from build123d import *

# Parameters (mm, degrees)
SKETCH1_R          = 16.5354
EXTRUDE1_DEPTH     = 53.848
CHAMFER1_SIZE      = 0.762
SKETCH6_R          = 15.6845
EXTRUDE2_DEPTH     = 5.969
SKETCH7_W          = 14.478
SKETCH7_H          = 10.31875
CUT_EXTRUDE4_DEPTH = 19.84248
HOLE1_D            = 5.0038
HOLE1_DEPTH        = 4.7498
CIRPATTERN1_COUNT  = 4


with BuildPart() as part:
    # Sketch1 → Extrude1 (new body)
    with BuildSketch(Plane.XY):
        Circle(SKETCH1_R)
    extrude(amount=EXTRUDE1_DEPTH)

    # Sketch2 → Cut-Revolve1 (revolve, cut)
    with BuildSketch(Plane(origin=(0, 0, 0), x_dir=(1, 0, 0), z_dir=(0, 1, 0)), mode=Mode.PRIVATE) as cut_revolve1_sk:
        Polygon((16.5354, -53.848), (16.5354, -39.9034), (15.2908, -41.148), (15.2908, -53.848), align=None)
    revolve(cut_revolve1_sk.sketch.rotate(Axis((0, 0, 0), (0, 0, 1)), 180), axis=Axis((0, 0, 0), (0, 0, 1)), mode=Mode.SUBTRACT)  # turned: the seam where the file's is

    # Sketch3 → Cut-Revolve2 (revolve, cut)
    with BuildSketch(Plane(origin=(0, 0, 0), x_dir=(1, 0, 0), z_dir=(0, 1, 0)), mode=Mode.PRIVATE) as cut_revolve2_sk:
        Polygon((15.2908, 0), (15.2908, -1.524), (16.5354, -2.7686), (16.5354, 0), align=None)
    revolve(cut_revolve2_sk.sketch.rotate(Axis((0, 0, 0), (0, 0, -1)), 180), axis=Axis((0, 0, 0), (0, 0, -1)), mode=Mode.SUBTRACT)  # turned: the seam where the file's is

    # S2D0002 → Cut-Revolve3 (revolve, cut)
    with BuildSketch(Plane(origin=(0, 0, 0), x_dir=(1, 0, 0), z_dir=(0, 1, 0))):
        Polygon((6.1849, -53.594), (9.525, -53.594), (9.525, -53.848), (0, -53.848), (0, -39.624), (4.9784, -39.624), (4.9784, -50.377393135), (5.642306865, -51.0413), align=None)
    revolve(axis=Axis((0, 0, 14.6685), (0, 0, -1)), mode=Mode.SUBTRACT)

    # Chamfer1
    chamfer1_edges = [part.edges().sort_by_distance(p)[0] for p in [
        (15.2908, 0, 53.848),
    ]]
    chamfer(chamfer1_edges, length=CHAMFER1_SIZE)

    # Sketch6 → Extrude2 (add)
    with BuildSketch(Plane(origin=(0, 0, 0), x_dir=(-1, 0, 0), z_dir=(0, 0, -1))):
        Circle(SKETCH6_R)
    extrude(amount=EXTRUDE2_DEPTH)

    # Sketch7 → Revolve1 (revolve)
    with BuildSketch(Plane(origin=(0, 0, 0), x_dir=(0, 0, -1), z_dir=(1, 0, 0)), mode=Mode.PRIVATE) as revolve1_sk:
        with Locations((13.208, -5.159375)):
            Rectangle(SKETCH7_W, SKETCH7_H)
    revolve(revolve1_sk.sketch.rotate(Axis((0, 0, 0), (0, 0, -1)), 270), axis=Axis((0, 0, 0), (0, 0, -1)))  # turned: the seam where the file's is

    # S2D0001 → Cut-Revolve5 (revolve, cut)
    with BuildSketch(Plane(origin=(0, 0, 0), x_dir=(1, 0, 0), z_dir=(0, 1, 0))):
        Polygon((3.2639, 18.511260017), (3.2639, 3.8608), (0, 3.8608), (0, 20.447), (4.3815, 20.447), align=None)
    revolve(axis=Axis((0, 0, 31.308359971), (0, 0, -1)), mode=Mode.SUBTRACT)

    # Sketch9 → Cut-Revolve6 (revolve, cut)
    with BuildSketch(Plane(origin=(0, 0, 0), x_dir=(0, -1, 0), z_dir=(1, 0, 0)), mode=Mode.PRIVATE) as cut_revolve6_sk:
        with BuildLine():
            Line((-10.31875, 13.0302), (-10.033, 13.7922))
            Line((-10.033, 13.7922), (-10.033, 19.431))
            ThreePointArc((-10.033, 19.431), (-9.932678675, 19.974796865), (-9.644922533, 20.447))
            Line((-9.644922533, 20.447), (-10.31875, 20.447))
            Line((-10.31875, 20.447), (-10.31875, 13.0302))
        make_face()
    revolve(cut_revolve6_sk.sketch.rotate(Axis((0, 0, -12.65936), (0, 0, -1)), 90), axis=Axis((0, 0, -12.65936), (0, 0, -1)), mode=Mode.SUBTRACT)  # turned: the seam where the file's is

    # Sketch13 → Cut-Extrude4 (cut, symmetric)
    with BuildSketch(Plane(origin=(0, 0, 0), x_dir=(1, 0, 0), z_dir=(0, 1, 0))):
        Polygon((8.5852, 20.447), (8.5852, 15.494), (10.033, 14.0462), (10.033, 20.447), align=None)
        Polygon((-8.5852, 20.447), (-8.5852, 15.494), (-10.033, 14.0462), (-10.033, 20.447), align=None)
    extrude(amount=CUT_EXTRUDE4_DEPTH, both=True, mode=Mode.SUBTRACT)

    # Hole1
    with Locations(Plane(origin=(-10.81222837, 10.81222837, 47.498), x_dir=(0.707106781, 0.707106781, 0), z_dir=(-0.707106781, 0.707106781, 0))):
        with Locations((0, 0)):
            hole1 = Hole(HOLE1_D / 2, depth=HOLE1_DEPTH)

    # CirPattern1: Hole1 ×4 about axis
    cirpattern1_axis = Axis((0, 0, 0), (0, 0, 1))
    for i in range(1, CIRPATTERN1_COUNT):
        add(hole1.rotate(cirpattern1_axis, i * 360 / CIRPATTERN1_COUNT), mode=Mode.SUBTRACT)


solid = part.part
Here's how the part is built. I have some questions about the finished solid (model axes, mm). A direction names the side the tool comes from. Round coordinates to 2 decimals unless told otherwise and drop trailing zeros. Write each loop counter-clockwise with the first axis right and the second up, starting at its lowest first coordinate (ties: lowest second). Pieces come first, ordered by that corner, then holes.
1. Suppose I cut it at B-B (z = 38). List the corners of the cut face in (x, y) for me.
2. For faces 4 (the cylindrical face through (-7.056, -13.566, 0.773)), 5 (the cylindrical face through (-14.125, 5.856, 47.201)), 6 (the flat face through (-10.2, -3.3, -5.969)), which set-ups out of +Z, -Z, +X, -X, +Y, -Y let a thin tool reach every point of the face, with its end or its side?
3. Suppose I cut it at D-D (z = -10). List the corners of the cut face in (x, y) for me.
4. Will these pins go through, and if not, where does the flat tip stop? pin 1 Ø12 at (x, z) = (9, -11.5) entering from -Y; pin 2 Ø6 at (x, y) = (9.5, -13) entering from -Z; pin 3 Ø3 at (x, y) = (2, 1) entering from +Z.
5. Suppose I cut it at C-C (x = 7). State how many separate pieces and enclosed holes the cut face has, and give its area (3 significant figures).
6. Suppose I cut it at A-A (z = 48.5). List the corners of the cut face in (x, y) for me, and give its area (3 significant figures).
7. If we mould it in two halves opening along X, with no side actions, what happens to faces 1 (the cylindrical face through (15.77, 4.97, 21.08)), 2 (the flat face through (9.14, -0.07, -14.94)), 3 (the cylindrical face through (4.749, -1.495, 45.076))? For each: released by +X, released by -X, zero draft, split by the parting line, or undercut.
8. I need wall thicknesses on L1, parallel to X at y = 9, z = 46; L2, parallel to X at y = 8.5, z = 49.5; L3, parallel to Y at x = 0, z = -12. Which ranges of each line are inside material? Lowest first, please.
Answer sheet:
1. outline: circle Ø33.07 at (0, 0)
2. face 4: none
2. face 5: +Z
2. face 6: -Z
3. outline: circle Ø20.64 at (0, 0); hole circle Ø6.53 at (0, 0)
4. pin 1: stops at y = -14.19
4. pin 2: stops at z = -5.97
4. pin 3: stops at z = 39.62
5. separate pieces: 1
5. enclosed holes: 2
5. area: 1,930 mm2
6. outline: (-12.31, -9.07) - (-9.07, -5.83) - (-5.83, -9.07) - (-9.07, -12.31) arc R15.29 ccw to (9.07, -12.31) - (5.83, -9.07) - (9.07, -5.83) - (12.31, -9.07) arc R15.29 ccw to (12.31, 9.07) - (9.07, 5.83) - (5.83, 9.07) - (9.07, 12.31) arc R15.29 ccw to (-9.07, 12.31) - (-5.83, 9.07) - (-9.07, 5.83) - (-12.31, 9.07) arc R15.29 ccw to start; hole circle Ø9.96 at (0, 0)
6. area: 571 mm2
7. face 1: split by the parting line
7. face 2: released by +X
7. face 3: undercut
8. L1: x = -12.36 to -11.83, -6.17 to 6.17, 11.83 to 12.36
8. L2: x = -12.71 to -10.62, -6.41 to 6.41, 10.62 to 12.71
8. L3: y = -10.32 to -3.26, 3.26 to 10.32
